Build history of the part. All positions in model axes, mm. Round coordinates to 2 decimals unless told otherwise and drop trailing zeros. Write each loop counter-clockwise with the first axis right and the second up, starting at its lowest first coordinate (ties: lowest second). Pieces come first, ordered by that corner, then holes. Notation, with made-up numbers: M 31,52.25 L 36,52.25 A14 cw 36,56.25 Z; hole C -35.5,-1 d10. An arc over 180 degrees is marked long. Write item = value, one per line. Start each with the question number.
Q1. Band-saw the part on D-D on x = -30. Write the cut outline in (y, z), plus the area to 3 significant figures.
Q2. Drop flat-ended pins along their axis: P1, Ø5.5, axis at x = 30, y = 0, coming from the +Z side; P2, Ø1.5, axis at y = -20, z = 8.5, coming from the -X side; P3, Ø4, axis at y = -23, z = 4, coming from the -X side (3 decimals); P4, Ø1, axis at y = 27.5, z = 6.5, coming from the +X side. Give the stop position or say it passes through.
Q3. Band-saw the part on C-C on z = 1.75. Write the cut outline in (x, y), plus the area to 3 significant figures.
Q4. Band-saw the part on B-B on y = 0. Write the cut outline in (x, z).
Q5. Probe L1, parallel to Y at x = 0, z = 7; L2, parallel to X at y = -2, z = 7; L3, parallel to Y at x = -30, z = 6.25. List the from-to ranges inside material, lowest first.
Q6. Band-saw the part on A-A on x = 0. Write the cut outline in (y, z), plus the area to 3 significant figures.
Q7. Pull direction Y, two halves, no side cores. Call faces 1 (the cylindrical face through (-33, 0, 5)), 2 (the cylindrical face through (-1.08, -4.88, 5.07)), 3 (the flat face through (12, 1, 0)), 4 (the cylindrical face through (-59.94, 2.64, 4.93)): released by +Y, released by -Y, zero draft, split by the parting line, or undercut.
```python
from build123d import *

# Parameters (mm, degrees)
SKETCH1_R           = 60
BOSS_EXTRUDE1_DEPTH = 10
SKETCH2_R           = 5
CUT_EXTRUDE1_DEPTH  = 10
SKETCH3_R           = 3
CUT_EXTRUDE2_DEPTH  = 10


with BuildPart() as part:
    # Sketch1 → Boss-Extrude1 (new body)
    with BuildSketch(Plane.XY):
        Circle(SKETCH1_R)
    extrude(amount=BOSS_EXTRUDE1_DEPTH)

    # Sketch2 → Cut-Extrude1 (cut)
    with BuildSketch(Plane.XY.offset(10)):
        Circle(SKETCH2_R)
    extrude(amount=-CUT_EXTRUDE1_DEPTH, mode=Mode.SUBTRACT)

    # Sketch3 → Cut-Extrude2 (cut)
    with BuildSketch(Plane.XY.offset(10)):
        with Locations((-30, 0)):
            Circle(SKETCH3_R)
        with Locations((30, 0)):
            Circle(SKETCH3_R)
    extrude(amount=-CUT_EXTRUDE2_DEPTH, mode=Mode.SUBTRACT)


solid = part.part
```
Conclusion:
q1.outline = M -51.96,0 L -3,0 L -3,10 L -51.96,10 Z; M 3,0 L 51.96,0 L 51.96,10 L 3,10 Z
q1.area = 979 mm^2
q2.P1 = through
q2.P2 = -56.83
q2.P3 = -56.205
q2.P4 = 53.58
q3.outline = C 0,0 d120; hole C -30,0 d6; hole C 0,0 d10; hole C 30,0 d6
q3.area = 11,200 mm^2
q4.outline = M -60,0 L -33,0 L -33,10 L -60,10 Z; M -27,0 L -5,0 L -5,10 L -27,10 Z; M 5,0 L 27,0 L 27,10 L 5,10 Z; M 33,0 L 60,0 L 60,10 L 33,10 Z
q5.L1 = -60 to -5, 5 to 60
q5.L2 = -59.97 to -32.24, -27.76 to -4.58, 4.58 to 27.76, 32.24 to 59.97
q5.L3 = -51.96 to -3, 3 to 51.96
q6.outline = M -60,0 L -5,0 L -5,10 L -60,10 Z; M 5,0 L 60,0 L 60,10 L 5,10 Z
q6.area = 1,100 mm^2
q7.face_1 = undercut
q7.face_2 = undercut
q7.face_3 = zero draft
q7.face_4 = split by the parting line
